Here's how the part is built. I have some questions about the finished solid (model axes, mm). Face numbers are marked on the shaded views. A direction names the side the tool comes from. Coordinates: 2 decimals unless noted, no trailing zeros. Order: outer loops, then holes, each group sorted by start corner. A loop starts at its lowest first (then second) coordinate and runs counter-clockwise, first axis right, second up. Notation, with made-up numbers: (87.25, 6.25) - (123.25, 6.25) arc R16 ccw to (123.25, 31.25) - close; hole circle Ø9 at (6, 16.5). An arc over 180 degrees is marked (long way). Answer in a Markdown table with one row per item. Add a question column.
Item 1: I want a section at D-D (x = 25.4). Please give me the cut outline in (y, z) (1 decimal).
Item 2: On a 3-axis mill with a long thin cutter (end or side, diameter ignored), from which of +Z, -Z, +X, -X, +Y, -Y can I reach the whole of each face in a straight line? I mean the marked faces 1 and 2. Say none if no direction works.
Item 3: Thinking about a two-plate mould opening in Y: for the marked faces 3, 4, 5 and 6, which applies, +Y half, -Y half, draft (parallel to the pull), parting line (faces both ways), or undercut?
Item 4: I want a section at B-B (y = -5.25). Please give me the cut outline in (x, z).
Item 5: I want a section at C-C (z = 35). Please give me the cut outline in (x, y), plus the area to 3 significant figures.
Item 6: If I drill on line 1 along Z through (x, y) = (33, -20.75); line 2 along Y through (x, z) = (22, 20); line 3 along Y through (x, z) = (38.5, 31), over which ranges is the centre line in solid material (lowest first)? Write a range as from..to.
Item 7: I want a section at A-A (x = 20). Please give me the cut outline in (y, z).
```python
from build123d import *

# Parameters (mm, degrees)
F1_DEPTH = 25.4
F3_DEPTH = 25.4
F4_SIZE  = 5.08


with BuildPart() as f1:
    # F0 (on Front) → F1 (new body)
    with BuildSketch(Plane.XZ):
        with BuildLine():
            Line((24.13, 18.0975), (0, 0))
            Line((0, 0), (50.8, 0))
            Line((50.8, 0), (50.8, 38.1))
            Line((50.8, 38.1), (26.67, 20.0025))
            ThreePointArc((26.67, 20.0025), (26.906035, 19.552012), (26.9875, 19.05))
            ThreePointArc((26.9875, 19.05), (25.902012, 17.543965), (24.13, 18.0975))
        make_face()
        with BuildLine():
            Line((0, 38.1), (0, 0))
            Line((0, 0), (24.13, 18.0975))
            ThreePointArc((24.13, 18.0975), (24.4475, 20.32), (26.67, 20.0025))
            Line((26.67, 20.0025), (50.8, 38.1))
            Line((50.8, 38.1), (0, 38.1))
        make_face()
    extrude(amount=F1_DEPTH)

    # F2 (on face) → F3 (cut)
    with BuildSketch(Plane.XY.offset(38.1)):
        Polygon((0, -6.35), (0, -19.05), (50.8, -25.4), (50.8, 0), align=None)
    extrude(amount=-F3_DEPTH, mode=Mode.SUBTRACT)

    # F4
    f4_edges = [f1.edges().sort_by_distance(p)[0] for p in [
        (50.8, -12.7, 0),
        (0, -12.7, 0),
    ]]
    chamfer(f4_edges, length=F4_SIZE)


solid = f1.part
```
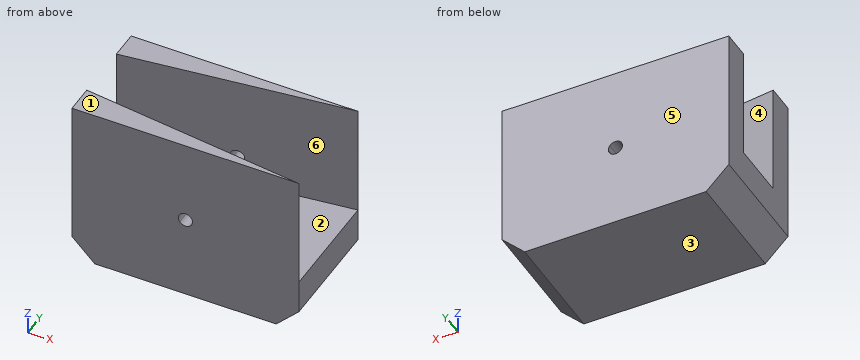
Values follow:
| question | item | result |
|---|---|---|
| 1 | outline | (-25.4, 0) - (0, 0) - (0, 17.5) - (-3.2, 17.5) - (-3.2, 12.7) - (-22.2, 12.7) - (-22.2, 17.5) - (-25.4, 17.5) - close; (-25.4, 20.6) - (-22.2, 20.6) - (-22.2, 38.1) - (-25.4, 38.1) - close; (-3.2, 20.6) - (0, 20.6) - (0, 38.1) - (-3.2, 38.1) - close |
| 2 | face 1 | +Z, +X, -X, +Y, -Y |
| 2 | face 2 | +Z, +X |
| 3 | face 3 | draft |
| 3 | face 4 | undercut |
| 3 | face 5 | +Y half |
| 3 | face 6 | undercut |
| 4 | outline | (0, 5.08) - (5.08, 0) - (45.72, 0) - (50.8, 5.08) - (50.8, 12.7) - (8.8, 12.7) - (8.8, 38.1) - (0, 38.1) - close |
| 5 | outline | (0, -25.4) - (50.8, -25.4) - (0, -19.05) - close; (0, -6.35) - (50.8, 0) - (0, 0) - close |
| 5 | area | 323 mm^2 |
| 6 | line 1 | z = 0..12.7 |
| 6 | line 2 | y = -25.4..-21.8, -3.6..0 |
| 6 | line 3 | y = -25.4..-23.86, -1.54..0 |
| 7 | outline | (-25.4, 0) - (0, 0) - (0, 38.1) - (-3.85, 38.1) - (-3.85, 12.7) - (-21.55, 12.7) - (-21.55, 38.1) - (-25.4, 38.1) - close |
